The listing builds one solid part. Answer for the finished solid, in the listing's coordinates (mm). Face numbers are marked on the shaded views. A direction names the side the tool comes from. Give positions to 0.01 mm unless a question says otherwise; leave off trailing zeros. Loops run counter-clockwise (first coordinate to the right, second up) from the corner with the lowest first, then second, coordinate; pieces in that order, holes last. Notation, with made-up numbers: M 49.25,32.5 L 96.25,32.5 A17 ccw 96.25,56.5 Z; hole C -6.75,32.25 d5. An arc over 180 degrees is marked long. One line per item, written item: value. Start each with the question number.
Q1. Consider L1, parallel to Y at x = -1.9, z = 21.25; L2, parallel to Z at x = -1.3, y = 22; L3, parallel to X at y = -22, z = 12.5. Determine where each line is inside the solid, lowest interval first.
Q2. A cutting plane is placed at D-D, the plane y = -17. State how many separate pieces and enclosed holes the cut face has, and give its area (3 significant figures).
Q3. A cutting plane is placed at C-C, the plane y = 14. Determine the outline of the cut face in (x, z) (3 decimals), and give its area (3 significant figures).
Q4. A cutting plane is placed at A-A, the plane z = 5. Determine the outline of the cut face in (x, y).
Q5. Flat-ended cylindrical pins translate along their axes: pin 1 (2 mm diameter, centred on y = 8, z = -17.5, fed in from +X); pin 2 (2 mm diameter, centred on x = 11.5, y = 2, fed in from +Z); pin 3 (6.5 mm diameter, centred on y = -20.5, z = 5, fed in from -X). Find the tip coordinate at first contact, or state that the pin passes through.
Q6. A cutting plane is placed at B-B, the plane x = 7.25. Determine the outline of the cut face in (y, z).
Q7. For the marked faces 1 and 2, determine the directions among +Z, -Z, +X, -X, +Y, -Y from which every point of the face is accessible in a straight line to the end or side of a thin tool.
from build123d import *

# Parameters (mm, degrees)
SKETCH1_W                       = 62
SKETCH1_H                       = 58
BOSS_EXTRUDE1_DEPTH             = 4
BOSS_EXTRUDE2_DEPTH             = 58
F_4_0MM_DOWEL_HOLE1_D           = 3.7
F_4_0MM_DOWEL_HOLE1_DEPTH       = 30
F_4_0MM_DOWEL_HOLE1_CSINK_D     = 3.71
F_4_0MM_DOWEL_HOLE1_CSINK_ANGLE = 90
F_4_0MM_DOWEL_HOLE1_TIP         = 1.111592145
F_6_0MM_DOWEL_HOLE1_AT_2_COUNT  = 2
F_6_0MM_DOWEL_HOLE1_AT_2_PITCH  = 32
F_6_0MM_DOWEL_HOLE1_AT_3_COUNT  = 2
F_6_0MM_DOWEL_HOLE1_AT_3_PITCH  = 42.544094772
SKETCH9_W                       = 9
SKETCH9_H                       = 62
BOSS_EXTRUDE3_DEPTH             = 4
SKETCH11_W                      = 9
SKETCH11_H                      = 58
BOSS_EXTRUDE4_DEPTH             = 4
F_4_0MM_DOWEL_HOLE2_AT_2_COUNT  = 2
F_4_0MM_DOWEL_HOLE2_AT_2_PITCH  = 32
SKETCH17_W                      = 8
SKETCH17_H                      = 30
CUT_EXTRUDE1_DEPTH              = 10
SKETCH20_W                      = 16
SKETCH20_H                      = 20
CUT_EXTRUDE2_DEPTH              = 10
CUT_EXTRUDE3_DEPTH              = 10
SKETCH22_R                      = 4
CUT_EXTRUDE4_DEPTH              = 10
SKETCH23_W                      = 12
SKETCH23_H                      = 20
CUT_EXTRUDE5_DEPTH              = 10
SKETCH24_W                      = 2.5
SKETCH24_H                      = 14
CUT_EXTRUDE6_DEPTH              = 10
MOVE_FACE2_BY                   = 2
SKETCH25_W                      = 12
SKETCH25_H                      = 12
BOSS_EXTRUDE5_DEPTH             = 4
EXTRUDE_THIN1_DEPTH             = 2
CHAMFER1_SIZE                   = 1.5
FILLET3_R                       = 1
SKETCH28_R                      = 4.5
CUT_EXTRUDE7_DEPTH              = 10
FILLET4_R                       = 2
EXTRUDE_THIN2_DEPTH             = 2
CUT_EXTRUDE9_DEPTH              = 0.8


with BuildPart() as part:
    # Sketch1 → Boss-Extrude1 (new body)
    with BuildSketch(Plane.YZ):
        Rectangle(SKETCH1_W, SKETCH1_H)
    extrude(amount=-BOSS_EXTRUDE1_DEPTH)

    # Sketch3 → Boss-Extrude2 (add)
    with BuildSketch(Plane.XY.offset(29)):
        Polygon((0, 31), (21, 31), (21, 28), (21, 18), (18, 18), (18, 28), (0, 28), align=None)
        Polygon((0, -31), (21, -31), (21, -28), (21, -18), (18, -18), (18, -28), (0, -28), align=None)
    extrude(amount=-BOSS_EXTRUDE2_DEPTH)

    # Ø4.0mm Dowel Hole1
    with Locations(Plane(origin=(0, 0, 0), x_dir=(0, 0, -1), z_dir=(1, 0, 0))):
        with Locations((3, -7), (3, 7), (16, 7)):
            CounterSinkHole(F_4_0MM_DOWEL_HOLE1_D / 2, F_4_0MM_DOWEL_HOLE1_CSINK_D / 2, depth=F_4_0MM_DOWEL_HOLE1_DEPTH, counter_sink_angle=F_4_0MM_DOWEL_HOLE1_CSINK_ANGLE)
            with Locations((0, 0, -(F_4_0MM_DOWEL_HOLE1_DEPTH + F_4_0MM_DOWEL_HOLE1_TIP / 2))):  # 118° drill point
                Cone(0, F_4_0MM_DOWEL_HOLE1_D / 2, F_4_0MM_DOWEL_HOLE1_TIP, mode=Mode.SUBTRACT)

    # Sketch7 → Ø6.0mm Dowel Hole1 (revolve, cut)
    with BuildSketch(Plane(origin=(0, 14, 21.25), x_dir=(0, 0, -1), z_dir=(0, 1, 0))):
        Polygon((0, 0), (0, 31.802581857), (3, 30), (3, 0.025), (3.025, 0), align=None)
    f_6_0mm_dowel_hole1 = revolve(axis=Axis((6.35, 14, 21.25), (-1, 0, 0)), mode=Mode.SUBTRACT)

    # Ø6.0mm Dowel Hole1 at 2: Ø6.0mm Dowel Hole1 ×2
    with Locations(*[(0, -i * F_6_0MM_DOWEL_HOLE1_AT_2_PITCH, 0) for i in range(1, F_6_0MM_DOWEL_HOLE1_AT_2_COUNT)]):
        add(f_6_0mm_dowel_hole1, mode=Mode.SUBTRACT)

    # Ø6.0mm Dowel Hole1 at 3: Ø6.0mm Dowel Hole1 ×2
    with Locations(*[Vector(0, -0.39958542051392815, -0.9166959647084235) * (i * F_6_0MM_DOWEL_HOLE1_AT_3_PITCH) for i in range(1, F_6_0MM_DOWEL_HOLE1_AT_3_COUNT)]):
        add(f_6_0mm_dowel_hole1, mode=Mode.SUBTRACT)

    # Sketch9 → Boss-Extrude3 (add)
    with BuildSketch(Plane(origin=(0, 0, -29), x_dir=(1, 0, 0), z_dir=(0, 0, -1))):
        with Locations((16.5, 0)):
            Rectangle(SKETCH9_W, SKETCH9_H)
    extrude(amount=-BOSS_EXTRUDE3_DEPTH)

    # Sketch11 → Boss-Extrude4 (add)
    with BuildSketch(Plane(origin=(0, -28, 0), x_dir=(-1, 0, 0), z_dir=(0, 1, 0))):
        with Locations((-16.5, 0)):
            Rectangle(SKETCH11_W, SKETCH11_H)
    boss_extrude4 = extrude(amount=BOSS_EXTRUDE4_DEPTH)

    # Mirror1: Boss-Extrude4 across plane
    add(boss_extrude4.mirror(Plane.ZX))

    # Sketch14 → Ø4.0mm Dowel Hole2 (revolve, cut)
    with BuildSketch(Plane(origin=(0, -10, 21.25), x_dir=(0, 0, -1), z_dir=(0, 1, 0))):
        Polygon((0, 0), (0, 31.201721238), (2, 30), (2, 0.025), (2.025, 0), align=None)
    f_4_0mm_dowel_hole2 = revolve(axis=Axis((6.35, -10, 21.25), (-1, 0, 0)), mode=Mode.SUBTRACT)

    # Ø4.0mm Dowel Hole2 at 2: Ø4.0mm Dowel Hole2 ×2
    with Locations(*[(0, i * F_4_0MM_DOWEL_HOLE2_AT_2_PITCH, 0) for i in range(1, F_4_0MM_DOWEL_HOLE2_AT_2_COUNT)]):
        add(f_4_0mm_dowel_hole2, mode=Mode.SUBTRACT)

    # Sketch17 → Cut-Extrude1 (cut)
    with BuildSketch(Plane.XZ.offset(31)):
        with Locations((4, 12)):
            Rectangle(SKETCH17_W, SKETCH17_H)
    cut_extrude1 = extrude(amount=-CUT_EXTRUDE1_DEPTH, mode=Mode.SUBTRACT)

    # Sketch20 → Cut-Extrude2 (cut)
    with BuildSketch(Plane.YZ):
        with Locations((-20, -19)):
            Rectangle(SKETCH20_W, SKETCH20_H)
    extrude(amount=-CUT_EXTRUDE2_DEPTH, mode=Mode.SUBTRACT)

    # Sketch21 → Cut-Extrude3 (cut)
    with BuildSketch(Plane.YZ):
        Polygon((-31, 10.25), (-21, 10.25), (-21, 7.75), (-21, 0.25), (-23.5, 0.25), (-23.5, 7.75), (-31, 7.75), align=None)
    cut_extrude3 = extrude(amount=-CUT_EXTRUDE3_DEPTH, mode=Mode.SUBTRACT)

    # Mirror2: Cut-Extrude1, Cut-Extrude3 across plane
    add(cut_extrude1.mirror(Plane.ZX), mode=Mode.SUBTRACT)
    add(cut_extrude3.mirror(Plane.ZX), mode=Mode.SUBTRACT)

    # Sketch22 → Cut-Extrude4 (cut)
    with BuildSketch(Plane.YZ):
        with Locations(Location((-3, -17.75, 0), (0, 0, 270))):
            Circle(SKETCH22_R)
    extrude(amount=-CUT_EXTRUDE4_DEPTH, mode=Mode.SUBTRACT)

    # Sketch23 → Cut-Extrude5 (cut)
    with BuildSketch(Plane.XZ.offset(31)):
        with Locations((2, -19)):
            Rectangle(SKETCH23_W, SKETCH23_H)
    extrude(amount=-CUT_EXTRUDE5_DEPTH, mode=Mode.SUBTRACT)

    # Sketch24 → Cut-Extrude6 (cut)
    with BuildSketch(Plane.XY.offset(-25)):
        with Locations((13.25, -17)):
            Rectangle(SKETCH24_W, SKETCH24_H)
    extrude(amount=-CUT_EXTRUDE6_DEPTH, mode=Mode.SUBTRACT)

    # Move Face2: a face moved outward by 2.0
    extrude(part.faces().sort_by_distance((9.4875, 31, -2.475))[0], amount=MOVE_FACE2_BY, dir=(0, 1, 0))

    # Sketch25 → Boss-Extrude5 (add)
    with BuildSketch(Plane.XY.offset(-25)):
        with Locations((6, 2)):
            Rectangle(SKETCH25_W, SKETCH25_H)
    extrude(amount=-BOSS_EXTRUDE5_DEPTH)

    # Sketch26 → Extrude-Thin1 (add)
    with BuildSketch(Plane(origin=(-4, 0, 0), x_dir=(0, -1, 0), z_dir=(-1, 0, 0))):
        Polygon((6.579571669, -23.95), (10.159143338, -17.75), (6.579571669, -11.55), (-0.579571669, -11.55), (-4.159143338, -17.75), (-0.579571669, -23.95), align=None)
        Polygon((6.0022214, -22.95), (9.0044428, -17.75), (6.0022214, -12.55), (-0.0022214, -12.55), (-3.0044428, -17.75), (-0.0022214, -22.95), align=None, mode=Mode.SUBTRACT)
    extrude(amount=EXTRUDE_THIN1_DEPTH)

    # Chamfer1
    chamfer1_edges = [part.edges().sort_by_distance(p)[0] for p in [
        (12, -10, -27),
    ]]
    chamfer(chamfer1_edges, length=CHAMFER1_SIZE)

    # Fillet3
    fillet3_edges = [part.edges().sort_by_distance(p)[0] for p in [
        (14, -10, -25),
        (6, -4, -25),
        (12, -6.25, -25),
        (12.75, -9.25, -25),
    ]]
    fillet(fillet3_edges, radius=FILLET3_R)

    # Sketch28 → Cut-Extrude7 (cut)
    with BuildSketch(Plane.YZ.offset(21)):
        with Locations((-18, 21.25)):
            Circle(SKETCH28_R)
    extrude(amount=-CUT_EXTRUDE7_DEPTH, mode=Mode.SUBTRACT)

    # Fillet4
    fillet4_edges = [part.edges().sort_by_distance(p)[0] for p in [
        (19.5, -18, 25.75),
        (19.5, -18, 16.75),
    ]]
    fillet(fillet4_edges, radius=FILLET4_R)

    # Sketch29 → Extrude-Thin2 (add)
    # profile 1 of 3: a face of its own
    with BuildSketch(Plane(origin=(-4, 0, 0), x_dir=(0, -1, 0), z_dir=(-1, 0, 0))):
        Polygon((-4.517393842, -7.3), (-2.034787685, -3), (-4.517393842, 1.3), (-9.482606158, 1.3), (-11.965212315, -3), (-9.482606158, -7.3), align=None)
        Polygon((-5.383419246, -5.8), (-3.766838493, -3), (-5.383419246, -0.2), (-8.616580754, -0.2), (-10.233161507, -3), (-8.616580754, -5.8), align=None, mode=Mode.SUBTRACT)
    # profile 2 of 3: a face of its own
    with BuildSketch(Plane(origin=(-4, 0, 0), x_dir=(0, -1, 0), z_dir=(-1, 0, 0))):
        Polygon((9.482606158, -7.3), (11.965212315, -3), (9.482606158, 1.3), (4.517393842, 1.3), (2.034787685, -3), (4.517393842, -7.3), align=None)
        Polygon((8.616580754, -5.8), (10.233161507, -3), (8.616580754, -0.2), (5.383419246, -0.2), (3.766838493, -3), (5.383419246, -5.8), align=None, mode=Mode.SUBTRACT)
    # profile 3 of 3: a face of its own
    with BuildSketch(Plane(origin=(-4, 0, 0), x_dir=(0, -1, 0), z_dir=(-1, 0, 0))):
        Polygon((-4.517393842, -20.3), (-2.034787685, -16), (-4.517393842, -11.7), (-9.482606158, -11.7), (-11.965212315, -16), (-9.482606158, -20.3), align=None)
        Polygon((-5.383419246, -18.8), (-3.766838493, -16), (-5.383419246, -13.2), (-8.616580754, -13.2), (-10.233161507, -16), (-8.616580754, -18.8), align=None, mode=Mode.SUBTRACT)
    extrude(amount=EXTRUDE_THIN2_DEPTH)

    # Sketch30 → Cut-Extrude9 (cut)
    with BuildSketch(Plane(origin=(-4, 0, 0), x_dir=(0, -1, 0), z_dir=(-1, 0, 0))):
        Polygon((-8.616580754, -0.2), (-10.233161507, -3), (-8.616580754, -5.8), (-5.383419246, -5.8), (-3.766838493, -3), (-5.383419246, -0.2), align=None)
        Polygon((5.383419246, -0.2), (3.766838493, -3), (5.383419246, -5.8), (8.616580754, -5.8), (10.233161507, -3), (8.616580754, -0.2), align=None)
        Polygon((-10.233161507, -16), (-8.616580754, -18.8), (-5.383419246, -18.8), (-3.766838493, -16), (-5.383419246, -13.2), (-8.616580754, -13.2), align=None)
    extrude(amount=-CUT_EXTRUDE9_DEPTH, mode=Mode.SUBTRACT)


solid = part.part
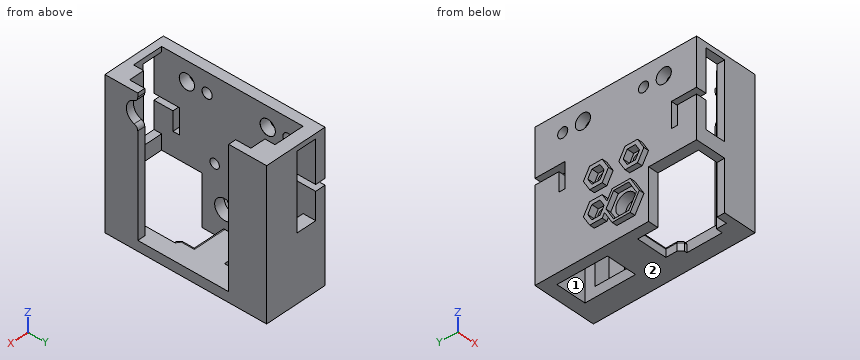
Answer block:
1. L1: -31 to -21, -15 to -12, -8 to 11, 17 to 20, 24 to 33
1. L2: -29 to 0.25, 10.25 to 19.25, 23.25 to 29
1. L3: -4 to 0, 18 to 21
2. separate pieces: 3
2. enclosed holes: 0
2. area: 155 mm^2
3. outline: M -4,-29 L 0,-29 L 0,18.225 L -0.025,18.25 L -4,18.25 Z; M -4,24.25 L -0.025,24.25 L 0,24.275 L 0,29 L -4,29 Z; M 12,-29 L 21,-29 L 21,-25 L 12,-25 Z
3. area: 244 mm^2
4. outline: M -4,-31 L 0,-31 L 0,-23.5 L -4,-23.5 Z; M -4,-21 L 0,-21 L 0,21 L -4,21 Z; M -4,23.5 L 0,23.5 L 0,33 L -4,33 Z; M 8,-31 L 21,-31 L 21,-18 L 18,-18 L 18,-24 L 12,-24 L 12,-28 L 8,-28 Z; M 8,28 L 12,28 L 12,24 L 18,24 L 18,18 L 21,18 L 21,33 L 8,33 Z
5. pin 1: x = 0
5. pin 2: z = -25
5. pin 3: x = -4
6. outline: M -31,-9 L -28,-9 L -28,-3 L -31,-3 Z; M -31,27 L -28,27 L -28,29 L -31,29 Z; M -4,-29 L 8,-29 L 8,-25 L -3,-25 A1 ccw -4,-26 Z; M 28,-29 L 33,-29 L 33,-3 L 28,-3 Z; M 28,27 L 33,27 L 33,29 L 28,29 Z
7. face 1: +Z, -Z
7. face 2: -Z, +X, -X, +Y, -Y
